from build123d import *

# Parameters (mm, degrees)
SKETCH_1_W          = 85
SKETCH_1_H          = 85
EXTRUDE_1_DEPTH     = 3
SKETCH_2_W          = 52.08
SKETCH_2_H          = 52.08
SKETCH_2_W_2        = 42.08
SKETCH_2_H_2        = 42.08
EXTRUDE_2_DEPTH     = 20
CHAMFER_1_SIZE      = 3
CHAMFER_2_SIZE      = 2
CHAMFER_3_SIZE      = 1
CHAMFER_4_SIZE      = 10
CHAMFER_5_SIZE      = 1
CUT_EXTRUDE_1_REACH = 124.389
SKETCH_3_W          = 8.5
SKETCH_3_H          = 9.566393395
SKETCH_3_H_2        = 3
SKETCH_3_H_3        = 9.81159244
CHAMFER_6_SIZE      = 1
CUT_EXTRUDE_2_DEPTH = 10
CUT_EXTRUDE_4_DEPTH = 59
SKETCH_6_R          = 1.65
CUT_EXTRUDE_5_DEPTH = 10


with BuildPart() as part:
    # 草图1 → 凸台-拉伸1 (new body)
    with BuildSketch(Plane(origin=(0, 0, 0), x_dir=(1, 0, 0), z_dir=(0, 1, 0))):
        with Locations((42.5, 42.5)):
            Rectangle(SKETCH_1_W, SKETCH_1_H)
    extrude(amount=EXTRUDE_1_DEPTH)

    # 草图2 → 凸台-拉伸2 (add)
    with BuildSketch(Plane(origin=(0, 3, 0), x_dir=(1, 0, 0), z_dir=(0, 1, 0))):
        with Locations((42.5, 42.5)):
            Rectangle(SKETCH_2_W, SKETCH_2_H)
        with Locations((42.5, 42.5)):
            Rectangle(SKETCH_2_W_2, SKETCH_2_H_2, mode=Mode.SUBTRACT)
    extrude(amount=EXTRUDE_2_DEPTH)

    # 倒角1
    chamfer_1_edges = [part.edges().sort_by_distance(p)[0] for p in [
        (16.46, 13, -68.54),
        (16.46, 13, -16.46),
        (68.54, 13, -16.46),
        (68.54, 13, -68.54),
        (63.54, 13, -63.54),
        (21.46, 13, -63.54),
        (21.46, 13, -21.46),
        (63.54, 13, -21.46),
    ]]
    chamfer(chamfer_1_edges, length=CHAMFER_1_SIZE)

    # 倒角2
    chamfer_2_edges = [part.edges().sort_by_distance(p)[0] for p in [
        (68.54, 3, -42.5),
        (42.5, 3, -16.46),
        (42.5, 3, -68.54),
        (16.46, 3, -42.5),
        (67.04, 3, -17.96),
        (67.04, 3, -67.04),
        (17.96, 3, -17.96),
        (17.96, 3, -67.04),
    ]]
    chamfer(chamfer_2_edges, length=CHAMFER_2_SIZE)

    # 倒角3
    chamfer_3_edges = [part.edges().sort_by_distance(p)[0] for p in [
        (68.54, 23, -42.5),
        (42.5, 23, -16.46),
        (16.46, 23, -42.5),
        (42.5, 23, -68.54),
        (63.54, 23, -42.5),
        (42.5, 23, -21.46),
        (21.46, 23, -42.5),
        (42.5, 23, -63.54),
        (17.96, 23, -67.04),
        (17.96, 23, -17.96),
        (67.04, 23, -67.04),
        (67.04, 23, -17.96),
        (62.04, 23, -22.96),
        (22.96, 23, -22.96),
        (62.04, 23, -62.04),
        (22.96, 23, -62.04),
    ]]
    chamfer(chamfer_3_edges, length=CHAMFER_3_SIZE)

    # 倒角4
    chamfer_4_edges = [part.edges().sort_by_distance(p)[0] for p in [
        (0, 1.5, -85),
        (85, 1.5, -85),
        (85, 1.5, 0),
        (0, 1.5, 0),
    ]]
    chamfer(chamfer_4_edges, length=CHAMFER_4_SIZE)

    # 倒角5
    chamfer_5_edges = [part.edges().sort_by_distance(p)[0] for p in [
        (0, 3, -42.5),
        (42.5, 3, -85),
        (42.5, 3, 0),
        (85, 3, -42.5),
        (80, 3, -5),
        (80, 3, -80),
        (5, 3, -5),
        (5, 3, -80),
    ]]
    chamfer(chamfer_5_edges, length=CHAMFER_5_SIZE)

    # 切除-拉伸1: up to this face of the body (flat: up to its plane)
    cut_extrude_1_end = Plane(part.part.faces().sort_by_distance((42.5, 3, -42.5))[0])
    # 草图3 → 切除-拉伸1 (cut, up to the picked face)
    with BuildSketch(Plane(origin=(0, 23, 0), x_dir=(1, 0, 0), z_dir=(0, 1, 0)), mode=Mode.PRIVATE) as cut_extrude_1_sk1:
        with Locations((46.75, 12.676803303)):
            Rectangle(SKETCH_3_W, SKETCH_3_H)
    cut_extrude_1_tool1 = split(extrude(cut_extrude_1_sk1.sketch, amount=-CUT_EXTRUDE_1_REACH, mode=Mode.PRIVATE), bisect_by=cut_extrude_1_end, keep=Keep.BOTH, mode=Mode.PRIVATE)
    # 草图3 → 切除-拉伸1 (cut, up to the picked face)
    with BuildSketch(Plane(origin=(0, 23, 0), x_dir=(1, 0, 0), z_dir=(0, 1, 0)), mode=Mode.PRIVATE) as cut_extrude_1_sk2:
        with Locations((46.75, 18.96)):
            Rectangle(SKETCH_3_W, SKETCH_3_H_2)
    cut_extrude_1_tool2 = split(extrude(cut_extrude_1_sk2.sketch, amount=-CUT_EXTRUDE_1_REACH, mode=Mode.PRIVATE), bisect_by=cut_extrude_1_end, keep=Keep.BOTH, mode=Mode.PRIVATE)
    # 草图3 → 切除-拉伸1 (cut, up to the picked face)
    with BuildSketch(Plane(origin=(0, 23, 0), x_dir=(1, 0, 0), z_dir=(0, 1, 0)), mode=Mode.PRIVATE) as cut_extrude_1_sk3:
        with Locations((46.75, 25.36579622)):
            Rectangle(SKETCH_3_W, SKETCH_3_H_3)
    cut_extrude_1_tool3 = split(extrude(cut_extrude_1_sk3.sketch, amount=-CUT_EXTRUDE_1_REACH, mode=Mode.PRIVATE), bisect_by=cut_extrude_1_end, keep=Keep.BOTH, mode=Mode.PRIVATE)
    # 草图3 → 切除-拉伸1 (cut, up to the picked face)
    with BuildSketch(Plane(origin=(0, 23, 0), x_dir=(1, 0, 0), z_dir=(0, 1, 0)), mode=Mode.PRIVATE) as cut_extrude_1_sk4:
        with Locations((38.25, 25.36579622)):
            Rectangle(SKETCH_3_W, SKETCH_3_H_3)
    cut_extrude_1_tool4 = split(extrude(cut_extrude_1_sk4.sketch, amount=-CUT_EXTRUDE_1_REACH, mode=Mode.PRIVATE), bisect_by=cut_extrude_1_end, keep=Keep.BOTH, mode=Mode.PRIVATE)
    # 草图3 → 切除-拉伸1 (cut, up to the picked face)
    with BuildSketch(Plane(origin=(0, 23, 0), x_dir=(1, 0, 0), z_dir=(0, 1, 0)), mode=Mode.PRIVATE) as cut_extrude_1_sk5:
        with Locations((38.25, 18.96)):
            Rectangle(SKETCH_3_W, SKETCH_3_H_2)
    cut_extrude_1_tool5 = split(extrude(cut_extrude_1_sk5.sketch, amount=-CUT_EXTRUDE_1_REACH, mode=Mode.PRIVATE), bisect_by=cut_extrude_1_end, keep=Keep.BOTH, mode=Mode.PRIVATE)
    # 草图3 → 切除-拉伸1 (cut, up to the picked face)
    with BuildSketch(Plane(origin=(0, 23, 0), x_dir=(1, 0, 0), z_dir=(0, 1, 0)), mode=Mode.PRIVATE) as cut_extrude_1_sk6:
        with Locations((38.25, 12.676803303)):
            Rectangle(SKETCH_3_W, SKETCH_3_H)
    cut_extrude_1_tool6 = split(extrude(cut_extrude_1_sk6.sketch, amount=-CUT_EXTRUDE_1_REACH, mode=Mode.PRIVATE), bisect_by=cut_extrude_1_end, keep=Keep.BOTH, mode=Mode.PRIVATE)
    add(cut_extrude_1_tool1.solids().sort_by(Axis((46.75, 23, -12.676803), (0, -1, 0)))[0], mode=Mode.SUBTRACT)
    add(cut_extrude_1_tool2.solids().sort_by(Axis((46.75, 23, -18.96), (0, -1, 0)))[0], mode=Mode.SUBTRACT)
    add(cut_extrude_1_tool3.solids().sort_by(Axis((46.75, 23, -25.365796), (0, -1, 0)))[0], mode=Mode.SUBTRACT)
    add(cut_extrude_1_tool4.solids().sort_by(Axis((38.25, 23, -25.365796), (0, -1, 0)))[0], mode=Mode.SUBTRACT)
    add(cut_extrude_1_tool5.solids().sort_by(Axis((38.25, 23, -18.96), (0, -1, 0)))[0], mode=Mode.SUBTRACT)
    add(cut_extrude_1_tool6.solids().sort_by(Axis((38.25, 23, -12.676803), (0, -1, 0)))[0], mode=Mode.SUBTRACT)

    # 倒角6
    chamfer_6_edges = [part.edges().sort_by_distance(p)[0] for p in [
        (34, 22.5, -16.96),
        (51, 22.5, -16.96),
        (51, 12.5, -21.46),
        (51, 22.5, -20.96),
        (51, 23, -18.96),
        (34, 12.5, -21.46),
        (34, 22.5, -20.96),
        (34, 4, -15.46),
        (34, 13.5, -16.46),
        (51, 4, -15.46),
        (51, 13.5, -16.46),
        (34, 23, -18.96),
    ]]
    chamfer(chamfer_6_edges, length=CHAMFER_6_SIZE)

    # 草图4 → 切除-拉伸2 (cut)
    with BuildSketch(Plane(origin=(0, 3, 0), x_dir=(1, 0, 0), z_dir=(0, 1, 0))):
        Polygon((25.288427125, 61.54), (22.874213562, 59.125786438), (22.874213562, 25.874213562), (25.288427125, 23.46), (33, 23.46), (52, 23.46), (59.711572875, 23.46), (61.54, 25.288427125), (61.54, 59.711572875), (59.711572875, 61.54), align=None)
    extrude(amount=-CUT_EXTRUDE_2_DEPTH, mode=Mode.SUBTRACT)

    # 草图5 → 切除-拉伸4 (cut)
    with BuildSketch(Plane.ZY.offset(-16.46)):
        Polygon((-63.54, 10.96), (-63.54, 7.96), (-61.58, 6), (-58.58, 6), align=None)
        Polygon((-63.54, 17.48), (-63.54, 14.48), (-55.06, 6), (-52.06, 6), align=None)
        Polygon((-45.54, 6), (-60.54, 21), (-63.54, 21), (-48.54, 6), align=None)
        Polygon((-40.02, 6), (-55.02, 21), (-58.02, 21), (-43.02, 6), align=None)
        Polygon((-34.5, 6), (-49.5, 21), (-52.5, 21), (-37.5, 6), align=None)
        Polygon((-28.98, 6), (-43.98, 21), (-46.98, 21), (-31.98, 6), align=None)
        Polygon((-23.46, 6), (-38.46, 21), (-41.46, 21), (-26.46, 6), align=None)
        Polygon((-21.46, 7.52), (-21.46, 10.52), (-31.94, 21), (-34.94, 21), align=None)
        Polygon((-21.46, 14.04), (-21.46, 17.04), (-25.42, 21), (-28.42, 21), align=None)
    extrude(amount=-CUT_EXTRUDE_4_DEPTH, mode=Mode.SUBTRACT)

    # 草图6 → 切除-拉伸5 (cut)
    with BuildSketch(Plane.XZ):
        with Locations(Location((75, -10, 0), (0, 0, 270))):
            Circle(SKETCH_6_R)
        with Locations(Location((75, -75, 0), (0, 0, 270))):
            Circle(SKETCH_6_R)
        with Locations(Location((10, -75, 0), (0, 0, 270))):
            Circle(SKETCH_6_R)
        with Locations(Location((10, -10, 0), (0, 0, 270))):
            Circle(SKETCH_6_R)
    extrude(amount=-CUT_EXTRUDE_5_DEPTH, mode=Mode.SUBTRACT)


solid = part.part
Could you check a few things on this model? Use its own coordinates, in mm. A direction names the side the tool comes from. Round coordinates to 2 decimals unless told otherwise and drop trailing zeros. Order: outer loops, then holes, each group sorted by start corner. A loop starts at its lowest first (then second) coordinate and runs counter-clockwise, first axis right, second up.
(1) If we mould it in two halves opening along Y, with no side actions, what happens to faces 1 (the flat face through (66, 6, -25)), 2 (the flat face through (80, 1, -80)), 3 (the flat face through (17.29, 4.01, -67.77))? For each: released by +Y, released by -Y, zero draft, split by the parting line, or undercut.
Response values:
face 1: undercut
face 2: zero draft
face 3: released by +Y
(2) Imagine slicing it at A-A (x = 53.5). Write out the boundary of the cut face in (y, z).
Response values:
outline: (0, -85) - (2, -85) - (3, -84) - (3, -70.54) - (5, -68.54) - (22, -68.54) - (23, -67.54) - (23, -64.54) - (22, -63.54) - (3, -63.54) - (3, -61.54) - (0, -61.54) - close; (0, -23.46) - (3, -23.46) - (3, -21.46) - (22, -21.46) - (23, -20.46) - (23, -17.46) - (22, -16.46) - (5, -16.46) - (3, -14.46) - (3, -1) - (2, 0) - (0, 0) - close
(3) Please list where these lines run through material, in increasing order: line 1 along X through (y, z) = (1.95, -75); line 2 along Z through (x, y) = (75, 1.6); line 3 along Z through (x, y) = (58, 8.25).
Response values:
line 1: x = 0 to 8.35, 11.65 to 73.35, 76.65 to 85
line 2: z = -85 to -76.65, -73.35 to -11.65, -8.35 to 0
line 3: z = -68.54 to -63.54, -21.46 to -16.46
(4) Which directions (+Z, -Z, +X, -X, +Y, -Y) give clear straight access to the entire face, cutting with the end or side of a thin tool? Please do faces 4 (the flat face through (22.94, 4.89, -62.02)), 5 (the flat face through (19.52, 15.69, -26.63)), 6 (the flat face through (68.54, 15, -42)), 7 (the flat face through (17.94, 13.38, -17.98)).
Response values:
face 4: +Y
face 5: +X, -X
face 6: +Z, -Z, +X, +Y
face 7: +Z, -X, +Y
(5) I'm going to push flat-ended pins straight in: pin 1 (3 mm diameter, centred on y = 10, z = -68, fed in from -X); pin 2 (5 mm diameter, centred on y = 16.5, z = -18.5, fed in from +X); pin 3 (9.5 mm diameter, centred on y = 12.5, z = -47.5, fed in from -X). Where does each tip first touch, or does it pass through?
Response values:
pin 1: stops at x = 17.42
pin 2: stops at x = 68.54
pin 3: stops at x = 16.46
